Work out the finished part from the listing and answer in its coordinate system (mm). A direction names the side the tool comes from. Give positions to 0.01 mm unless a question says otherwise; leave off trailing zeros. Loops run counter-clockwise (first coordinate to the right, second up) from the corner with the lowest first, then second, coordinate; pieces in that order, holes last. Notation, with made-up numbers: M 65.25,-2.5 L 89.25,-2.5 A27 ccw 89.25,31.5 Z; hole C -1.75,35.25 d9. An arc over 180 degrees is marked long. Write item = value, one per line. Start each with the question number.
1. Section A-A on x = 75 is taken. Determine the outline of the cut face in (y, z), plus the area to 4 significant figures.
2. Section C-C on x = 2.5 is taken. Determine the outline of the cut face in (y, z) (3 decimals).
3. Section B-B on y = 2.5 is taken. Determine the outline of the cut face in (x, z).
4. Section D-D on z = -3.5 is taken. Give the number of separate pieces and of enclosed holes in the cut face, plus the area to 3 significant figures.
5. The mould has two halves that part along Y. Classify faces 1 (the face through (26.5, 68, -5)), 2 (the face through (95, 41, -8)): released by +Y, released by -Y, zero draft, split by the parting line, or undercut.
6. For faces 3 (the face through (2, 22.25, -7)), 4 (the face through (52.5, 20, -3)), 5 (the face through (9.079, 10.345, -1.929)), 6 (the face through (14.5, 68, -5)), determine the directions among +Z, -Z, +X, -X, +Y, -Y from which every point of the face is accessible in a straight line to the end or side of a thin tool.
7. Flat-ended cylindrical pins translate along their axes: pin 1 Ø1 at (y, z) = (22, -6) entering from -X; pin 2 Ø1.4 at (x, y) = (10, 60) entering from -Z; pin 3 Ø8 at (x, y) = (80, 49) entering from -Z; pin 4 Ø1 at (x, y) = (43.5, 31) entering from -Z. Find the tip coordinate at first contact, or state that the pin passes through.
8. Consider L1, parallel to Y at x = 10, z = -0.5; L2, parallel to Y at x = 94.5, z = -6; L3, parallel to X at y = 47, z = -2.75. Determine where each line is inside the solid, lowest interval first. Write a range as [from, to].
```python
from build123d import *

# Parameters (mm, degrees)
SKETCH1_W           = 100
SKETCH1_H           = 70
SKETCH1_R           = 1.5
SKETCH1_R_2         = 1.25
SKETCH1_R_3         = 1
BOSS_EXTRUDE6_DEPTH = 2
BOSS_EXTRUDE7_START = -7
SKETCH1_16_W        = 100
SKETCH1_16_H        = 70
SKETCH1_16_R        = 1.5
SKETCH1_16_W_2      = 90
SKETCH1_16_H_2      = 60
SKETCH1_16_W_3      = 8
SKETCH1_16_H_3      = 7
SKETCH1_16_R_2      = 1.75
SKETCH1_16_W_4      = 7.5
SKETCH1_16_H_4      = 8
SKETCH1_16_W_5      = 8.5
SKETCH1_16_H_5      = 8.5
SKETCH1_16_R_3      = 1.25
SKETCH1_16_R_4      = 0.625
BOSS_EXTRUDE7_DEPTH = 7
SKETCH1_18_W        = 10
SKETCH1_18_H        = 6
BOSS_EXTRUDE8_DEPTH = 5.5
CUT_EXTRUDE2_START  = -5.75
SKETCH1_19_R        = 1.25
SKETCH1_19_R_2      = 0.625
CUT_EXTRUDE2_DEPTH  = 5.75
BOSS_EXTRUDE9_START = -13.25
SKETCH1_20_W        = 100
SKETCH1_20_H        = 70
SKETCH1_20_R        = 1.5
SKETCH1_20_W_2      = 90
SKETCH1_20_H_2      = 60
BOSS_EXTRUDE9_DEPTH = 13.25
SKETCH4_W           = 10.25
SKETCH4_H           = 11.5
CUT_EXTRUDE3_DEPTH  = 5
SKETCH5_W           = 3.75
SKETCH5_H           = 8.5
CUT_EXTRUDE4_DEPTH  = 5
SKETCH6_W           = 11
SKETCH6_H           = 7
CUT_EXTRUDE5_DEPTH  = 5


with BuildPart() as part:
    # Sketch1 → Boss-Extrude6 (new body)
    with BuildSketch(Plane.XY):
        with Locations((50, 35)):
            Rectangle(SKETCH1_W, SKETCH1_H)
        with Locations((2.5, 2.5)):
            Circle(SKETCH1_R, mode=Mode.SUBTRACT)
        with Locations((2.5, 67.5)):
            Circle(SKETCH1_R, mode=Mode.SUBTRACT)
        with Locations((97.5, 67.5)):
            Circle(SKETCH1_R, mode=Mode.SUBTRACT)
        with Locations((97.5, 2.5)):
            Circle(SKETCH1_R, mode=Mode.SUBTRACT)
        with Locations((10, 9.5)):
            Circle(SKETCH1_R_2, mode=Mode.SUBTRACT)
        with Locations((10, 60)):
            Circle(SKETCH1_R_2, mode=Mode.SUBTRACT)
        with Locations((91, 41.5)):
            Circle(SKETCH1_R_2, mode=Mode.SUBTRACT)
        with Locations((91, 9.5)):
            Circle(SKETCH1_R_2, mode=Mode.SUBTRACT)
        with Locations((19.5, 12.5)):
            Circle(SKETCH1_R_3, mode=Mode.SUBTRACT)
        with Locations((75, 55)):
            Circle(SKETCH1_R_3, mode=Mode.SUBTRACT)
        with Locations((75, 25)):
            Circle(SKETCH1_R_3, mode=Mode.SUBTRACT)
    extrude(amount=BOSS_EXTRUDE6_DEPTH)

    # Sketch1<16> → Boss-Extrude7 (add)
    # profile 1 of 13: a face of its own
    with BuildSketch(Plane.XY.offset(BOSS_EXTRUDE7_START)):
        with Locations((50, 35)):
            Rectangle(SKETCH1_16_W, SKETCH1_16_H)
        with Locations((97.5, 2.5)):
            Circle(SKETCH1_16_R, mode=Mode.SUBTRACT)
        with Locations((97.5, 67.5)):
            Circle(SKETCH1_16_R, mode=Mode.SUBTRACT)
        with Locations((2.5, 67.5)):
            Circle(SKETCH1_16_R, mode=Mode.SUBTRACT)
        with Locations((2.5, 2.5)):
            Circle(SKETCH1_16_R, mode=Mode.SUBTRACT)
        with Locations((50, 35)):
            Rectangle(SKETCH1_16_W_2, SKETCH1_16_H_2, mode=Mode.SUBTRACT)
    # profile 2 of 13: a face of its own
    with BuildSketch(Plane.XY.offset(BOSS_EXTRUDE7_START)):
        with Locations((9, 8.5)):
            Rectangle(SKETCH1_16_W_3, SKETCH1_16_H_3)
        with Locations((10, 9.5)):
            Circle(SKETCH1_16_R_2, mode=Mode.SUBTRACT)
    # profile 3 of 13: a face of its own
    with BuildSketch(Plane.XY.offset(BOSS_EXTRUDE7_START)):
        with Locations((91.25, 9)):
            Rectangle(SKETCH1_16_W_4, SKETCH1_16_H_4)
        with Locations((91, 9.5)):
            Circle(SKETCH1_16_R_2, mode=Mode.SUBTRACT)
    # profile 4 of 13: a face of its own
    with BuildSketch(Plane.XY.offset(BOSS_EXTRUDE7_START)):
        with Locations((91.25, 41.5)):
            Rectangle(SKETCH1_16_W_4, SKETCH1_16_H_3)
        with Locations((91, 41.5)):
            Circle(SKETCH1_16_R_2, mode=Mode.SUBTRACT)
    # profile 5 of 13: a face of its own
    with BuildSketch(Plane.XY.offset(BOSS_EXTRUDE7_START)):
        with Locations((9.25, 60.75)):
            Rectangle(SKETCH1_16_W_5, SKETCH1_16_H_5)
        with Locations((10, 60)):
            Circle(SKETCH1_16_R_2, mode=Mode.SUBTRACT)
    # profile 6 of 13: a face of its own
    with BuildSketch(Plane.XY.offset(BOSS_EXTRUDE7_START)):
        with Locations((10, 60)):
            Circle(SKETCH1_16_R_2)
        with Locations((10, 60)):
            Circle(SKETCH1_16_R_3, mode=Mode.SUBTRACT)
    # profile 7 of 13: a face of its own
    with BuildSketch(Plane.XY.offset(BOSS_EXTRUDE7_START)):
        with Locations((10, 60)):
            Circle(SKETCH1_16_R_3)
        with Locations((10, 60)):
            Circle(SKETCH1_16_R_4, mode=Mode.SUBTRACT)
    # profile 8 of 13: a face of its own
    with BuildSketch(Plane.XY.offset(BOSS_EXTRUDE7_START)):
        with Locations((10, 9.5)):
            Circle(SKETCH1_16_R_2)
        with Locations((10, 9.5)):
            Circle(SKETCH1_16_R_3, mode=Mode.SUBTRACT)
    # profile 9 of 13: a face of its own
    with BuildSketch(Plane.XY.offset(BOSS_EXTRUDE7_START)):
        with Locations((10, 9.5)):
            Circle(SKETCH1_16_R_3)
        with Locations((10, 9.5)):
            Circle(SKETCH1_16_R_4, mode=Mode.SUBTRACT)
    # profile 10 of 13: a face of its own
    with BuildSketch(Plane.XY.offset(BOSS_EXTRUDE7_START)):
        with Locations((91, 9.5)):
            Circle(SKETCH1_16_R_2)
        with Locations((91, 9.5)):
            Circle(SKETCH1_16_R_3, mode=Mode.SUBTRACT)
    # profile 11 of 13: a face of its own
    with BuildSketch(Plane.XY.offset(BOSS_EXTRUDE7_START)):
        with Locations((91, 9.5)):
            Circle(SKETCH1_16_R_3)
        with Locations((91, 9.5)):
            Circle(SKETCH1_16_R_4, mode=Mode.SUBTRACT)
    # profile 12 of 13: a face of its own
    with BuildSketch(Plane.XY.offset(BOSS_EXTRUDE7_START)):
        with Locations((91, 41.5)):
            Circle(SKETCH1_16_R_2)
        with Locations((91, 41.5)):
            Circle(SKETCH1_16_R_3, mode=Mode.SUBTRACT)
    # profile 13 of 13: a face of its own
    with BuildSketch(Plane.XY.offset(BOSS_EXTRUDE7_START)):
        with Locations((91, 41.5)):
            Circle(SKETCH1_16_R_3)
        with Locations((91, 41.5)):
            Circle(SKETCH1_16_R_4, mode=Mode.SUBTRACT)
    extrude(amount=BOSS_EXTRUDE7_DEPTH)

    # Sketch1<18> → Boss-Extrude8 (add)
    with BuildSketch(Plane.XY):
        Polygon((19.5, 32.5), (19.5, 57.5), (70.5, 57.5), (70.5, 27.5), (52.5, 27.5), (52.5, 12.5), (32.5, 12.5), (32.5, 32.5), align=None)
        with Locations((49.5, 49)):
            Rectangle(SKETCH1_18_W, SKETCH1_18_H, mode=Mode.SUBTRACT)
    extrude(amount=-BOSS_EXTRUDE8_DEPTH)

    # Sketch1<19> → Cut-Extrude2 (cut)
    # profile 1 of 4: a face of its own
    with BuildSketch(Plane.XY.offset(CUT_EXTRUDE2_START)):
        with Locations((10, 60)):
            Circle(SKETCH1_19_R)
        with Locations((10, 60)):
            Circle(SKETCH1_19_R_2, mode=Mode.SUBTRACT)
    # profile 2 of 4: a face of its own
    with BuildSketch(Plane.XY.offset(CUT_EXTRUDE2_START)):
        with Locations((10, 9.5)):
            Circle(SKETCH1_19_R)
        with Locations((10, 9.5)):
            Circle(SKETCH1_19_R_2, mode=Mode.SUBTRACT)
    # profile 3 of 4: a face of its own
    with BuildSketch(Plane.XY.offset(CUT_EXTRUDE2_START)):
        with Locations((91, 9.5)):
            Circle(SKETCH1_19_R)
        with Locations((91, 9.5)):
            Circle(SKETCH1_19_R_2, mode=Mode.SUBTRACT)
    # profile 4 of 4: a face of its own
    with BuildSketch(Plane.XY.offset(CUT_EXTRUDE2_START)):
        with Locations((91, 41.5)):
            Circle(SKETCH1_19_R)
        with Locations((91, 41.5)):
            Circle(SKETCH1_19_R_2, mode=Mode.SUBTRACT)
    extrude(amount=CUT_EXTRUDE2_DEPTH, mode=Mode.SUBTRACT)

    # Sketch1<20> → Boss-Extrude9 (add)
    with BuildSketch(Plane.XY.offset(BOSS_EXTRUDE9_START)):
        with Locations((50, 35)):
            Rectangle(SKETCH1_20_W, SKETCH1_20_H)
        with Locations((97.5, 2.5)):
            Circle(SKETCH1_20_R, mode=Mode.SUBTRACT)
        with Locations((97.5, 67.5)):
            Circle(SKETCH1_20_R, mode=Mode.SUBTRACT)
        with Locations((2.5, 67.5)):
            Circle(SKETCH1_20_R, mode=Mode.SUBTRACT)
        with Locations((2.5, 2.5)):
            Circle(SKETCH1_20_R, mode=Mode.SUBTRACT)
        with Locations((50, 35)):
            Rectangle(SKETCH1_20_W_2, SKETCH1_20_H_2, mode=Mode.SUBTRACT)
    extrude(amount=BOSS_EXTRUDE9_DEPTH)

    # Sketch4 → Cut-Extrude3 (cut)
    with BuildSketch(Plane(origin=(100, 0, 0), x_dir=(0, 0, -1), z_dir=(1, 0, 0))):
        with Locations((6.125, 31.25)):
            Rectangle(SKETCH4_W, SKETCH4_H)
    extrude(amount=-CUT_EXTRUDE3_DEPTH, mode=Mode.SUBTRACT)

    # Sketch5 → Cut-Extrude4 (cut)
    with BuildSketch(Plane.ZY):
        with Locations((-6.5, 18)):
            Rectangle(SKETCH5_W, SKETCH5_H)
    extrude(amount=-CUT_EXTRUDE4_DEPTH, mode=Mode.SUBTRACT)

    # Sketch6 → Cut-Extrude5 (cut)
    with BuildSketch(Plane(origin=(0, 70, 0), x_dir=(1, 0, 0), z_dir=(0, 1, 0))):
        with Locations((20, 5.5)):
            Rectangle(SKETCH6_W, SKETCH6_H)
        with Locations((32, 5.5)):
            Rectangle(SKETCH6_W, SKETCH6_H)
    extrude(amount=-CUT_EXTRUDE5_DEPTH, mode=Mode.SUBTRACT)


solid = part.part
```
Verdict:
q1.outline = M 0,-13.25 L 5,-13.25 L 5,0 L 24,0 L 24,2 L 0,2 Z; M 26,0 L 54,0 L 54,2 L 26,2 Z; M 56,0 L 65,0 L 65,-13.25 L 70,-13.25 L 70,2 L 56,2 Z
q1.area = 264.5 mm2
q2.outline = M 0,-13.25 L 1,-13.25 L 1,2 L 0,2 Z; M 4,-13.25 L 66,-13.25 L 66,2 L 4,2 Z; M 69,-13.25 L 70,-13.25 L 70,2 L 69,2 Z; hole M 13.75,-8.375 L 22.25,-8.375 L 22.25,-4.625 L 13.75,-4.625 Z
q3.outline = M 0,-13.25 L 1,-13.25 L 1,2 L 0,2 Z; M 4,-13.25 L 96,-13.25 L 96,2 L 4,2 Z; M 99,-13.25 L 100,-13.25 L 100,2 L 99,2 Z
q4.separate_pieces = 4
q4.enclosed_holes = 9
q4.area = 3,330 mm2
q5.face_1 = zero draft
q5.face_2 = undercut
q6.face_3 = -X
q6.face_4 = -Z
q6.face_5 = +Z
q6.face_6 = +Y
q7.pin_1 = 0
q7.pin_2 = -7
q7.pin_3 = 0
q7.pin_4 = -5.5
q8.L1 = [0, 8.25], [10.75, 12], [56.5, 58.75], [61.25, 70]
q8.L2 = [0, 13], [38, 45], [65, 70]
q8.L3 = [0, 5], [19.5, 44.5], [54.5, 70.5], [95, 100]
